```python
from build123d import *

# Parameters (mm, degrees)
REVOLUTION_ANGLE   = -360
SKETCH006_R        = 10
POCKET_DEPTH       = 261.517738
POLARPATTERN_COUNT = 5
SKETCH007_R        = 9
PAD_DEPTH          = 20
POCKET001_DEPTH    = 5
SKETCH009_R        = 2
POCKET002_DEPTH    = 37.001


with BuildPart() as part:
    # Sketch004 → Revolution (revolve, symmetric)
    with BuildSketch(Plane.XZ) as revolution_sk:
        with BuildLine():
            Line((0, 0), (0, 7))
            Line((0, 7), (5, 7))
            add(Edge.make_bspline(
                [(5, 7), (20.98773, 16.664236), (32, 30)],
                knots=[0, 0, 0, 1, 1, 1], degree=2))
            Line((32, 30), (35, 30))
            Line((35, 30), (35, -30))
            Line((35, -30), (32, -30))
            Line((32, -30), (32, 0))
            Line((32, 0), (0, 0))
        make_face()
    revolve(axis=Axis((0, 0, 0), (0, 0, 1)), revolution_arc=REVOLUTION_ANGLE / 2)
    revolve(revolution_sk.sketch, axis=Axis((0, 0, 0), (0, 0, -1)), revolution_arc=REVOLUTION_ANGLE / 2)

    # Sketch006 → Pocket (cut, through all)
    with BuildSketch(Plane.XY):
        with Locations((0, 20)):
            Circle(SKETCH006_R)
    pocket = extrude(amount=POCKET_DEPTH, mode=Mode.SUBTRACT)

    # PolarPattern: Pocket ×5 about axis
    polarpattern_axis = Axis((0, 0, 0), (0, 0, 1))
    for i in range(1, POLARPATTERN_COUNT):
        add(pocket.rotate(polarpattern_axis, i * 360 / POLARPATTERN_COUNT), mode=Mode.SUBTRACT)

    # Sketch007 → Pad (join)
    with BuildSketch(Plane.XY):
        Circle(SKETCH007_R)
    extrude(amount=-PAD_DEPTH)

    # Sketch008 (on Face14 of Pad) → Pocket001 (cut)
    with BuildSketch(Plane(origin=(0, 0, -20), x_dir=(1, 0, 0), z_dir=(0, 0, -1))):
        Polygon((6.495191, -3.75), (6.495191, 3.75), (0, 7.5), (-6.495191, 3.75), (-6.495191, -3.75), (0, -7.5), align=None)
    extrude(amount=-POCKET001_DEPTH, mode=Mode.SUBTRACT)

    # Sketch009 (on Face1 of Pocket001) → Pocket002 (cut, through all)
    with BuildSketch(Plane(origin=(0, 0, 7), x_dir=(-1, 0, 0), z_dir=(0, 0, 1))):
        Circle(SKETCH009_R)
    extrude(amount=-POCKET002_DEPTH, mode=Mode.SUBTRACT)


solid = part.part
```
Here's how the part is built. I have some questions about the finished solid (model axes, mm). A direction names the side the tool comes from. Give positions to 0.01 mm unless a question says otherwise; leave off trailing zeros. Write each question's results on one line, items separated by ' | '.
Item 1: Suppose I cut it at A-A on x = -4. Give the number of separate pieces and of enclosed holes in the cut face, plus the area to 3 significant figures.
Output:
separate pieces: 3 | enclosed holes: 0 | area: 1,110 mm^2
Item 2: If I drill on L1, parallel to Y at x = -1, z = -23.5; L2, parallel to X at y = 6.5, z = -4.5; L3, parallel to X at y = 13.5, z = 15.5, over which ranges is the centre line in solid material (lowest first)?
Output:
L1: y = -34.99 to -31.98, 31.98 to 34.99 | L2: x = -34.39 to -31.33, -6.22 to 6.22, 31.33 to 34.39 | L3: x = -32.29 to -25.83, -12.21 to -10.69, 10.69 to 12.21, 25.83 to 32.29
Item 3: On a 3-axis mill with a long thin cutter (end or side, diameter ignored), from which of +Z, -Z, +X, -X, +Y, -Y can I reach the whole of each face in a straight line? I mean faces 3 (the face through (1, 2, -15)), 4 (the face through (-15.4, -28.4, 30)), 5 (the face through (-2.2, 0.1, 7)). Say none if no direction works.
Output:
face 3: -Z | face 4: +Z, +X, -X, +Y, -Y | face 5: +Z
Item 4: We'd pull the mould along X, two halves only. Please class faces 1 (the face through (15.4, -28.4, -30)), 2 (the face through (-1.172, 8.923, -9.86)): pulls with the +X half, pulls with the -X half, needs draft (parallel to the pull), parting line crosses it, or undercut.
Output:
face 1: needs draft | face 2: undercut
Item 5: For pin 1 Ø5 at (x, y) = (-1, -2) entering from +Z; pin 2 Ø1.5 at (y, z) = (-7, 7.5) entering from -X; pin 3 Ø18 at (x, y) = (-19.02, 6.18) entering from -Z; pin 4 Ø5 at (x, z) = (27.5, 20) entering from +Y, each with a flat end and sliding along its axis, tell me the tip position at first contact or that it passes through.
Output:
pin 1: stops at z = 7 | pin 2: stops at x = -34.44 | pin 3: passes through | pin 4: stops at y = 24.49
